The drawing under review shows one solid part. Ordinate dimensions are in mm from its lowest x, y, z. A direction names the side the tool comes from. Give positions to 0.01 mm unless a question says otherwise; leave off trailing zeros. Write each loop counter-clockwise with the first axis right and the second up, starting at its lowest first coordinate (ties: lowest second). Pieces come first, ordered by that corner, then holes. Notation, with made-up numbers: (-39, 23.5) -> (13, 23.5) arc R28 ccw to (13, 42.5) -> close; hole circle Ø4 at (40, 6). An arc over 180 degrees is marked (long way). Write item = value, one per line.
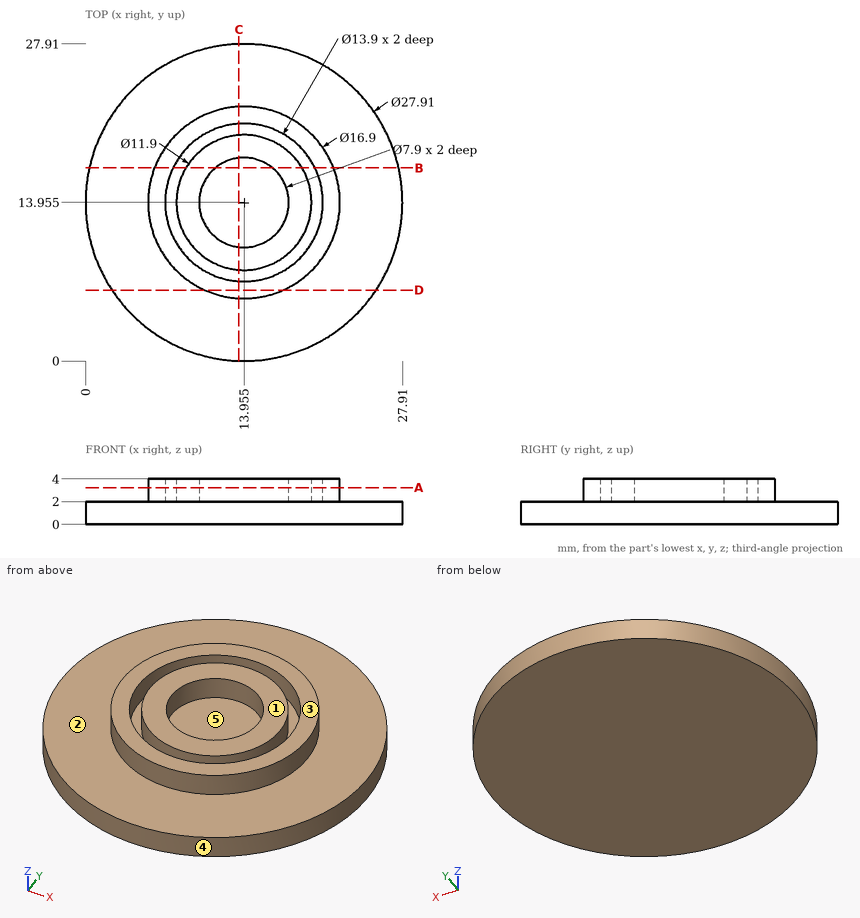
(1) The part is to be moulded in two halves that separate along X. For the marked faces 3, 4 and 5, say which applies: released by +X, released by -X, zero draft, split by the parting line, or undercut.
Answers below:
face_3 = zero draft
face_4 = split by the parting line
face_5 = undercut
(2) For pin 1 (14 mm diameter, centred on x = 13, y = 15.5, fed in from +Z); pin 2 (1 mm diameter, centred on y = 12, z = 2, fed in from -X); pin 3 (2 mm diameter, centred on x = 4.5, y = 3.5, fed in from +Z); pin 4 (1.5 mm diameter, centred on x = 20.5, z = 3, fed in from +Y) (1 decimal), all flat-tipped, find the tip position at first contact; note any pin that passes through.
Answers below:
pin_1 = 4
pin_2 = 0.08
pin_3 = 2
pin_4 = 20.1
(3) Take a section at B-B (y = 17). Write out the cut boundary in (x, z).
Answers below:
outline = (0.34, 0) -> (27.57, 0) -> (27.57, 2) -> (21.84, 2) -> (21.84, 4) -> (20.2, 4) -> (20.2, 2) -> (19.07, 2) -> (19.07, 4) -> (16.47, 4) -> (16.47, 2) -> (11.44, 2) -> (11.44, 4) -> (8.84, 4) -> (8.84, 2) -> (7.71, 2) -> (7.71, 4) -> (6.07, 4) -> (6.07, 2) -> (0.34, 2) -> close
(4) Take a section at A-A (z = 3.25). Write out the cut boundary in (x, y) (3 decimals), plus the area to 3 significant figures.
Answers below:
outline = circle Ø16.9 at (13.955, 13.955); circle Ø11.9 at (13.955, 13.955); hole circle Ø13.9 at (13.955, 13.955); hole circle Ø7.9 at (13.955, 13.955)
area = 135 mm^2
(5) To check wall thickness, follow probe 1 along X at (y, z) = (9.75, 3.55) (1 decimal); probe 2 along Z at (x, y) = (21.25, 25); probe 3 along X at (y, z) = (14.75, 2.85). State the ranges of each line that lie inside material, in increasing order.
Answers below:
probe_1 = 6.6 to 8.4, 9.7 to 18.2, 19.5 to 21.3
probe_2 = 0 to 2
probe_3 = 5.54 to 7.05, 8.06 to 10.09, 17.82 to 19.85, 20.86 to 22.37
(6) Tool access review of the marked faces 1 and 2: name each direction out of +Z, -Z, +X, -X, +Y, -Y from which nothing blocks a thin tool from reaching the whole face with its end or side.
Answers below:
face_1 = +Z, +X, -X, +Y, -Y
face_2 = +Z
(7) Take a section at C-C (x = 13.5). Write out the cut boundary in (y, z).
Answers below:
outline = (0.01, 0) -> (27.9, 0) -> (27.9, 2) -> (22.39, 2) -> (22.39, 4) -> (20.89, 4) -> (20.89, 2) -> (19.89, 2) -> (19.89, 4) -> (17.88, 4) -> (17.88, 2) -> (10.03, 2) -> (10.03, 4) -> (8.02, 4) -> (8.02, 2) -> (7.02, 2) -> (7.02, 4) -> (5.52, 4) -> (5.52, 2) -> (0.01, 2) -> close
(8) Take a section at D-D (y = 6.25). Write out the cut boundary in (x, z).
Answers below:
outline = (2.32, 0) -> (25.59, 0) -> (25.59, 2) -> (17.42, 2) -> (17.42, 4) -> (10.49, 4) -> (10.49, 2) -> (2.32, 2) -> close
